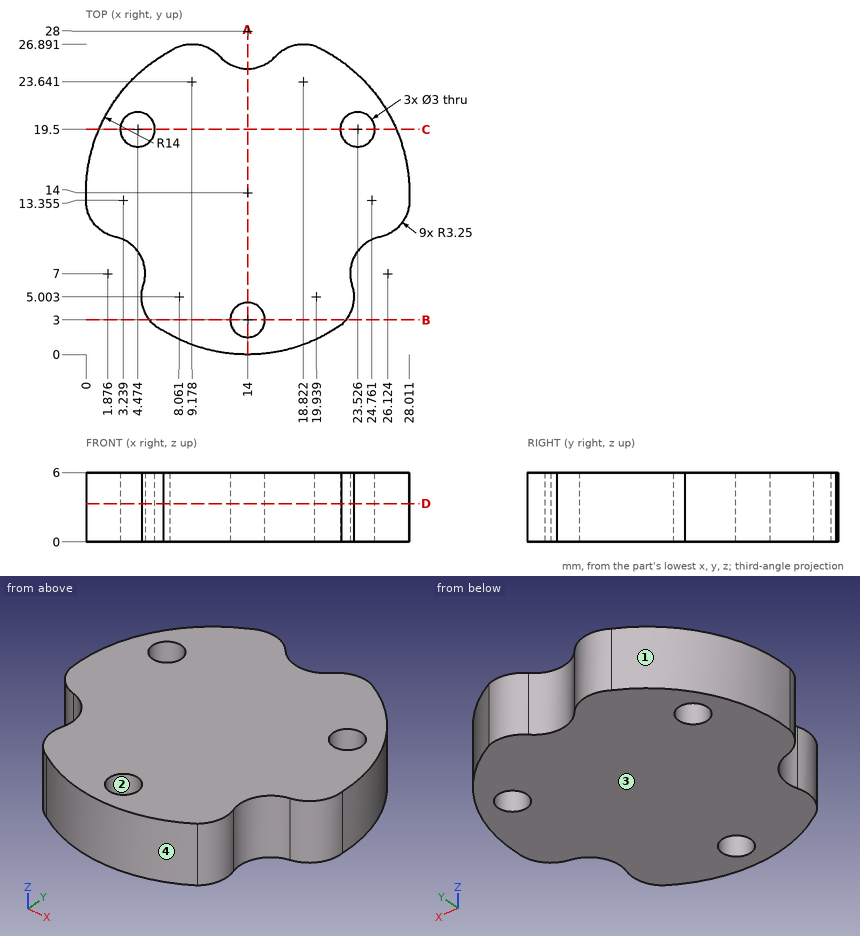
Drawing for the job (mm, zero at the part's lowest x, y, z). Give positions to 0.01 mm unless a question says otherwise; leave off trailing zeros. Order: outer loops, then holes, each group sorted by start corner. A loop starts at its lowest first (then second) coordinate and runs counter-clockwise, first axis right, second up. Notation, with made-up numbers: (80, 85) - (116, 85) arc R26 cw to (116, 104) - close; hole circle Ø1 at (82.25, -29.75). An arc over 180 degrees is marked (long way). Write item = value, one per line. Start each with the question number.
1. Cut at B-B, the plane y = 3. List the corners of the cut face in (x, z).
2. Probe line 1 along X through (y, z) = (2.75, 3.2); line 2 along X through (y, z) = (18.5, 1.6) (1 decimal); line 3 along Y through (x, z) = (3.5, 1.5) (1 decimal). List the from-to ranges inside material, lowest first.
3. Cut at A-A, the plane x = 14. List the corners of the cut face in (y, z).
4. Cut at D-D, the plane z = 3.3. State how many separate pieces and enclosed holes the cut face has, and give its area (3 significant figures).
5. Two-plate mould, pull along X, no slides. Class the marked faces 1, 2, 3 and 4: pulls with the +X half, pulls with the -X half, needs draft (parallel to the pull), parting line crosses it, or undercut.
6. Cut at C-C, the plane y = 19.5. List the corners of the cut face in (x, z) (1 decimal).
7. Drop flat-ended pins along their axis: P1, Ø2, axis at x = 3, y = 22, coming from the -Z side; P2, Ø1.5, axis at x = 9, z = 4.5, coming from the -Y side. Give the stop position or say it passes through.
Taken from the geometry:
q1.outline = (5.5, 0) - (12.5, 0) - (12.5, 6) - (5.5, 6) - close; (15.5, 0) - (22.5, 0) - (22.5, 6) - (15.5, 6) - close
q2.line_1 = 5.72 to 12.52, 15.48 to 22.28
q2.line_2 = 0.7 to 3.4, 5.6 to 22.4, 24.6 to 27.3
q2.line_3 = 9.8 to 18.4, 20.6 to 23.3
q3.outline = (0, 0) - (1.5, 0) - (1.5, 6) - (0, 6) - close; (4.5, 0) - (24.75, 0) - (24.75, 6) - (4.5, 6) - close
q4.separate_pieces = 1
q4.enclosed_holes = 3
q4.area = 539 mm²
q5.face_1 = pulls with the -X half
q5.face_2 = undercut
q5.face_3 = needs draft
q5.face_4 = parting line crosses it
q6.outline = (1.1, 0) - (3, 0) - (3, 6) - (1.1, 6) - close; (6, 0) - (22, 0) - (22, 6) - (6, 6) - close; (25, 0) - (26.9, 0) - (26.9, 6) - (25, 6) - close
q7.P1 = 0
q7.P2 = 0.66
